Autodesk Inventor part; units mm, degrees
ref_plane "YZ Plane" through (0, 0, 0) normal (1, 0, 0) x (0, 1, 0)
ref_plane "XZ Plane" through (0, 0, 0) normal (0, 1, 0) x (-1, 0, 0)
ref_plane "XY Plane" through (0, 0, 0) normal (0, 0, 1) x (1, 0, 0)
sketch "Esquisse1" plane through (0, 0, 0) normal (0, 0, 1) x (1, 0, 0)
  line L0 (0, 0) -> (52, 0) construction
  line L1 (0, 0) -> (27.5772, 27.5772) construction
  circle A0 centre (27.5772, 27.5772) radius 2
  circle A1 centre (0, 0) radius 2
  line L2 (0, 0) -> (0, -8) construction
  line L3 (0, 0) -> (-5.6569, 5.6569) construction
  line L4 (68.2971, -8) -> (-19.3137, -8)
  line L5 (27.5772, 27.5772) -> (27.5772, 35.5772) construction
  line L6 (-19.3137, -8) -> (24.2635, 35.5772)
  line L7 (24.2635, 35.5772) -> (68.2971, 35.5772)
  line L8 (27.5772, 27.5772) -> (49, 27.5772) construction
  line L9 (27.5772, 27.5772) -> (55.1548, 4.4368) construction
  line L10 (27.5772, 27.5772) -> (36.2548, 37.9188) construction
  line L11 (36.2548, 37.9188) -> (41.2341, 33.7406) construction
  line L12 (41.2341, 33.7406) -> (47.3624, 28.5983) construction
  line L13 (47.3624, 28.5983) -> (53.4908, 23.456) construction
  line L14 (53.4908, 23.456) -> (59.6192, 18.3137) construction
  line L15 (55.1548, 4.4368) -> (60.2971, 10.5652) construction
  circle A2 centre (41.2341, 33.7406) radius 1 construction
  circle A3 centre (47.3624, 28.5983) radius 1
  circle A4 centre (53.4908, 23.456) radius 1
  circle A5 centre (59.6192, 18.3137) radius 1
  circle A6 centre (60.2971, 10.5652) radius 1
  circle A7 centre (23.8788, 13.0574) radius 1 construction
  circle A8 centre (30.0072, 7.9151) radius 1
  circle A9 centre (36.1355, 2.7728) radius 1
  circle A10 centre (42.2639, -2.3695) radius 1
  circle A11 centre (50.0125, -1.6915) radius 1
  line L16 (60.2971, 10.5652) -> (68.2971, 10.5652) construction
  line L17 (68.2971, 35.5772) -> (68.2971, -8)
  dimension "d39" = 39
  dimension "d41" = 4
  dimension "d44" = 8
  dimension "d64" = 8
  dimension "d80" = 45
  dimension "d82" = 8
  dimension "d101" = 36
  dimension "d102" = 40
  dimension "d103" = 13.5
  dimension "d104" = 6.5
  dimension "d105" = 8
  dimension "d106" = 8
  dimension "d107" = 8
  dimension "d108" = 8
  dimension "d109" = 2
  dimension "d110" = 8
extrude "Extrusion15" add sketch "Esquisse1" along normal blind 12
sketch "Esquisse13" plane through (0, 0, 12) normal (0, 0, 1) x (1, 0, 0)
  circle A0 centre (0, 0) radius 2
  circle A1 centre (27.5772, 27.5772) radius 2
  line L0 (68.2971, -8) -> (68.2971, 35.5772)
  line L1 (68.2971, 35.5772) -> (24.2635, 35.5772)
  line L2 (24.2635, 35.5772) -> (-19.3137, -8)
  circle A2 centre (27.5772, 27.5772) radius 12 construction
  line L3 (39.5772, 35.5772) -> (39.5772, 27.5772)
  line L4 (0, 0) -> (0, 8) construction
  line L5 (-4.4796, 6.8341) -> (30.5997, 15.964)
  arc A3 (30.5997, 15.964) -> (39.5772, 27.5772) centre (27.5772, 27.5772) ccw
  dimension "d128" = 24
  dimension "d129" = 8
extrude "Extrusion16" cut sketch "Esquisse13" against normal blind 7 contours L3 A3 L5 L2 L1
sketch "Esquisse14" plane through (0, 0, 12) normal (0, 0, 1) x (1, 0, 0)
  line L0 (-19.3137, -8) -> (68.2971, -8)
  circle A0 centre (0, 0) radius 2
  line L1 (4.0415, 0) -> (2.0207, -3.5)
  line L2 (2.0207, -3.5) -> (-2.0207, -3.5)
  line L3 (-2.0207, -3.5) -> (-4.0415, 0)
  line L4 (-4.0415, 0) -> (-2.0207, 3.5)
  line L5 (-2.0207, 3.5) -> (2.0207, 3.5)
  line L6 (2.0207, 3.5) -> (4.0415, 0)
  line L7 (2.0207, 3.5) -> (2.0207, -3.5) construction
  dimension "d132" = 7
sketch "Esquisse15" plane through (0, 0, 5) normal (0, 0, 1) x (1, 0, 0)
  circle A0 centre (27.5772, 27.5772) radius 2
  arc A1 (30.5997, 15.964) -> (39.5772, 27.5772) centre (27.5772, 27.5772) ccw
  line L0 (31.6186, 27.5772) -> (29.5979, 24.0772)
  line L1 (29.5979, 24.0772) -> (25.5564, 24.0772)
  line L2 (25.5564, 24.0772) -> (23.5357, 27.5772)
  line L3 (23.5357, 27.5772) -> (25.5564, 31.0772)
  line L4 (25.5564, 31.0772) -> (29.5979, 31.0772)
  line L5 (29.5979, 31.0772) -> (31.6186, 27.5772)
  line L6 (-19.3137, -8) -> (68.2971, -8)
  line L7 (-2.0207, 3.5) -> (2.0207, 3.5)
  point P0 (0, 0)
extrude "Extrusion17" cut sketch "Esquisse14" against normal blind 3
extrude "Extrusion18" cut sketch "Esquisse15" against normal blind 3
fillet "Congé8" radius 8 1 edges at (-19.3137, -8, 6)
fillet "Congé9" radius 8 1 edges at (24.2635, 35.5772, 2.5)
fillet "Congé10" radius 8 1 edges at (39.5772, 35.5772, 8.5)
chamfer "Chanfrein1" distance 15 angle 45 1 edges at (68.2971, 35.5772, 6)
chamfer "Chanfrein2" distance 15 angle 45 1 edges at (68.2971, -8, 6)
fillet "Congé12" radius 10 1 edges at (53.2971, -8, 6)
fillet "Congé13" radius 10 1 edges at (68.2971, 7, 6)
fillet "Congé14" radius 10 1 edges at (68.2971, 20.5772, 6)
fillet "Congé15" radius 10 1 edges at (53.2971, 35.5772, 6)
properties part number "joint1+ax12imprint+v2"
Design review of the part built by this model. Coordinates are the model's own, in mm. A direction names the side the tool comes from. Coordinates: 2 decimals unless noted, no trailing zeros. Order: outer loops, then holes, each group sorted by start corner. A loop starts at its lowest first (then second) coordinate and runs counter-clockwise, first axis right, second up. Notation, with made-up numbers: (80.25, 36) - (99.25, 36) arc R22 ccw to (99.25, 45) - close; hole circle Ø9 at (33, -25.5). An arc over 180 degrees is marked (long way). One line per question, with ' | ' between items.
Q1. Consider section C-C, the plane y = 14.5. Give the boundary of the cut face in (x, z), then the cut area to 3 significant figures.
Answer key:
outline: (3.19, 0) - (68.3, 0) - (68.3, 12) - (24.97, 12) - (24.97, 5) - (3.19, 5) - close | area: 629 mm2
Q2. For faces 4 (the flat face through (28, 31.077, 4)), 5 (the cylindrical face through (49.013, -1.735, 5.916)), 6 (the flat face through (21, 21, 5)), list the 3-axis set-ups (+Z, -Z, +X, -X, +Y, -Y) from which the entire face can be reached by the end or side of a thin tool; tool diameter is ignored.
Answer key:
face 4: +Z | face 5: +Z, -Z | face 6: +Z, -X, +Y
Q3. Consider section D-D, the plane x = 38.5. Give the boundary of the cut face in (y, z), then the cut area to 3 significant figures.
Answer key:
outline: (-8, 0) - (35.58, 0) - (35.58, 5) - (22.61, 5) - (22.61, 12) - (-8, 12) - close | area: 432 mm2
Q4. The part is to be moulded in two halves that separate along X. For faces 1 (the flat face through (25, -8, 6)), 2 (the flat face through (0, 3.5, 11)), 3 (the flat face through (7.939, 19.252, 3.249)), say which applies: +X half, -X half, draft (parallel to the pull), parting line (faces both ways), or undercut.
Answer key:
face 1: draft | face 2: undercut | face 3: -X half
Q5. Clearance check with flat-ended pins moving along their axes: pin 1 Ø6 at (x, y) = (11, 20) entering from +Z; pin 2 Ø1 at (x, z) = (28, 6.5) entering from +Y; pin 3 Ø3 at (y, z) = (24, 5.5) entering from -X. State where each tip first meets the part, or that it passes through.
Answer key:
pin 1: stops at z = 5 | pin 2: stops at y = 15.42 | pin 3: stops at x = 11.27
Q6. To check wall thickness, follow line 1 along X through (y, z) = (29, 2.25); line 2 along X through (y, z) = (28, 1.5); line 3 along Y through (x, z) = (46.5, 2.25). State the ranges of each line that lie inside material, in increasing order.
Answer key:
line 1: x = 17.69 to 24.36, 30.8 to 46.45, 48.28 to 59.87 | line 2: x = 16.69 to 25.62, 29.53 to 46.56, 48.16 to 60.87 | line 3: y = -8 to 28.09, 29.1 to 35.58
Q7. Consider section A-A, the plane z = 8. Give the number of separate pieces and of enclosed holes in the cut face, then the cut area to 3 significant figures.
Answer key:
separate pieces: 1 | enclosed holes: 9 | area: 1,920 mm2
